Build history of the part. All positions in model axes, mm. Face numbers are marked on the shaded views. A direction names the side the tool comes from. Coordinates: 2 decimals unless noted, no trailing zeros. Write each loop counter-clockwise with the first axis right and the second up, starting at its lowest first coordinate (ties: lowest second). Pieces come first, ordered by that corner, then holes.
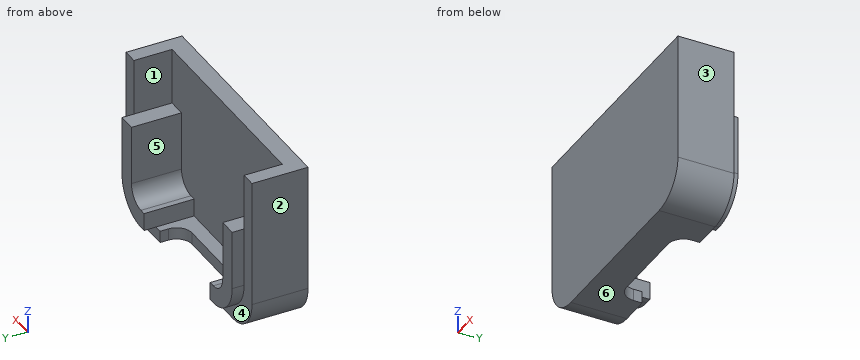
```python
from build123d import *

# Parameters (mm, degrees)
BOSS_EXTRUDE1_DEPTH = 1.5
BOSS_EXTRUDE2_START = 3.2
BOSS_EXTRUDE2_DEPTH = 3.2
BOSS_EXTRUDE3_START = 4.2
BOSS_EXTRUDE3_DEPTH = 4.2
CUT_EXTRUDE1_DEPTH  = 24.43560539


with BuildPart() as part:
    # Sketch1 → Boss-Extrude1 (new body)
    with BuildSketch(Plane(origin=(0, 0, 0), x_dir=(1, 0, 0), z_dir=(0, 1, 0))):
        with BuildLine():
            Line((-1.5, 20.46), (-1.5, 9.7))
            Line((-1.5, 9.7), (18.5, 9.7))
            Line((18.5, 9.7), (18.5, 20.46))
            ThreePointArc((18.5, 20.46), (17.621320344, 22.581320344), (15.5, 23.46))
            Line((15.5, 23.46), (1.5, 23.46))
            ThreePointArc((1.5, 23.46), (-0.621320344, 22.581320344), (-1.5, 20.46))
        make_face()
    extrude(amount=-BOSS_EXTRUDE1_DEPTH)

    # Sketch3 → Boss-Extrude2 (add)
    with BuildSketch(Plane(origin=(0, 0, 0), x_dir=(1, 0, 0), z_dir=(0, 1, 0)).offset(BOSS_EXTRUDE2_START)):
        with BuildLine():
            Line((2.75, 22.46), (14.25, 22.46))
            ThreePointArc((14.25, 22.46), (16.371320344, 21.581320344), (17.25, 19.46))
            Line((17.25, 19.46), (17.25, 9.7))
            Line((17.25, 9.7), (18.5, 9.7))
            Line((18.5, 9.7), (18.5, 20.46))
            ThreePointArc((18.5, 20.46), (17.621320344, 22.581320344), (15.5, 23.46))
            Line((15.5, 23.46), (1.5, 23.46))
            ThreePointArc((1.5, 23.46), (-0.621320344, 22.581320344), (-1.5, 20.46))
            Line((-1.5, 20.46), (-1.5, 9.7))
            Line((-1.5, 9.7), (-0.25, 9.7))
            Line((-0.25, 9.7), (-0.25, 19.46))
            ThreePointArc((-0.25, 19.46), (0.628679656, 21.581320344), (2.75, 22.46))
        make_face()
    extrude(amount=-BOSS_EXTRUDE2_DEPTH)

    # Sketch2 → Boss-Extrude3 (add)
    with BuildSketch(Plane(origin=(0, 0, 0), x_dir=(1, 0, 0), z_dir=(0, 1, 0)).offset(BOSS_EXTRUDE3_START)):
        with BuildLine():
            Line((2.75, 20.96), (3.25, 20.96))
            Line((3.25, 20.96), (3.25, 22.46))
            Line((3.25, 22.46), (2.75, 22.46))
            ThreePointArc((2.75, 22.46), (0.628679656, 21.581320344), (-0.25, 19.46))
            Line((-0.25, 19.46), (-0.25, 14.46))
            Line((-0.25, 14.46), (1.25, 14.46))
            Line((1.25, 14.46), (1.25, 19.46))
            ThreePointArc((1.25, 19.46), (1.689339828, 20.520660172), (2.75, 20.96))
        make_face()
        with BuildLine():
            Line((17.25, 19.46), (17.25, 14.46))
            Line((17.25, 14.46), (15.75, 14.46))
            Line((15.75, 14.46), (15.75, 19.46))
            ThreePointArc((15.75, 19.46), (15.310660172, 20.520660172), (14.25, 20.96))
            Line((14.25, 20.96), (13.75, 20.96))
            Line((13.75, 20.96), (13.75, 22.46))
            Line((13.75, 22.46), (14.25, 22.46))
            ThreePointArc((14.25, 22.46), (16.371320344, 21.581320344), (17.25, 19.46))
        make_face()
    extrude(amount=-BOSS_EXTRUDE3_DEPTH)

    # Sketch5 → Cut-Extrude1 (cut, through all)
    with BuildSketch(Plane(origin=(0, 0, -23.46), x_dir=(-1, 0, 0), z_dir=(0, 0, -1))):
        with BuildLine():
            Line((-13.1, 3.2), (-3.9, 3.2))
            Line((-3.9, 3.2), (-3.9, 2.5))
            ThreePointArc((-3.9, 2.5), (-4.280761184, 1.580761184), (-5.2, 1.2))
            Line((-5.2, 1.2), (-11.8, 1.2))
            ThreePointArc((-11.8, 1.2), (-12.719238816, 1.580761184), (-13.1, 2.5))
            Line((-13.1, 2.5), (-13.1, 3.2))
        make_face()
    extrude(amount=-CUT_EXTRUDE1_DEPTH, mode=Mode.SUBTRACT)


solid = part.part
```
1. Probe line 1 along X through (y, z) = (0.05, -16); line 2 along X through (y, z) = (1.85, -13); line 3 along Y through (x, z) = (10, -14). List the from-to ranges inside material, lowest first.
Computed values:
line 1: x = -1.5 to 1.25, 15.75 to 18.5
line 2: x = -1.5 to -0.25, 17.25 to 18.5
line 3: y = -1.5 to 0
2. Flat gauge pins, fed straight in: pin 1 (0.5 mm diameter, centred on x = 8.5, z = -23, fed in from +Y); pin 2 (1.2 mm diameter, centred on y = 2, z = -22, fed in from +X); pin 3 (1 mm diameter, centred on x = 11, z = -12, fed in from +Y). Where does each tip first touch, or does it go through?
Computed values:
pin 1: stops at y = 1.2
pin 2: stops at x = 18.35
pin 3: stops at y = 0
3. Saw through at C-C on x = 5.5. List the corners of the cut face in (y, z).
Computed values:
outline: (-1.5, -23.46) - (1.2, -23.46) - (1.2, -22.46) - (0, -22.46) - (0, -9.7) - (-1.5, -9.7) - close
4. Saw through at A-A on y = 2.8. List the corners of the cut face in (x, z).
Computed values:
outline: (-1.5, -20.46) arc R3 ccw to (1.5, -23.46) - (3.9, -23.46) - (3.9, -22.46) - (3.25, -22.46) - (3.25, -20.96) - (2.75, -20.96) arc R1.5 cw to (1.25, -19.46) - (1.25, -14.46) - (-0.25, -14.46) - (-0.25, -9.7) - (-1.5, -9.7) - close; (13.1, -23.46) - (15.5, -23.46) arc R3 ccw to (18.5, -20.46) - (18.5, -9.7) - (17.25, -9.7) - (17.25, -14.46) - (15.75, -14.46) - (15.75, -19.46) arc R1.5 cw to (14.25, -20.96) - (13.75, -20.96) - (13.75, -22.46) - (13.1, -22.46) - close
5. Saw through at D-D on y = 0.65. List the corners of the cut face in (x, z).
Computed values:
outline: (-1.5, -20.46) arc R3 ccw to (1.5, -23.46) - (15.5, -23.46) arc R3 ccw to (18.5, -20.46) - (18.5, -9.7) - (17.25, -9.7) - (17.25, -14.46) - (15.75, -14.46) - (15.75, -19.46) arc R1.5 cw to (14.25, -20.96) - (13.75, -20.96) - (13.75, -22.46) - (3.25, -22.46) - (3.25, -20.96) - (2.75, -20.96) arc R1.5 cw to (1.25, -19.46) - (1.25, -14.46) - (-0.25, -14.46) - (-0.25, -9.7) - (-1.5, -9.7) - close
6. Saw through at B-B on z = -19.25. List the corners of the cut face in (x, y), plus the area to 3 significant figures.
Computed values:
outline: (-1.5, -1.5) - (18.5, -1.5) - (18.5, 3.2) - (17.25, 3.2) - (17.25, 4.2) - (15.75, 4.2) - (15.75, 0) - (1.25, 0) - (1.25, 4.2) - (-0.25, 4.2) - (-0.25, 3.2) - (-1.5, 3.2) - close
area: 50.6 mm2
7. 3-axis set-ups, long thin cutter, end or side, ignore diameter. For the marked faces 4, 5 and 6: which of +Z, -Z, +X, -X, +Y, -Y reach the whole face in a straight line?
Computed values:
face 4: -Z, -X, +Y
face 5: +Z, +Y
face 6: -Z, +X, -X, +Y, -Y
8. Mould opens along X. For the marked faces 1, 2 and 3 say: +X half, -X half, draft (parallel to the pull), parting line (faces both ways), or undercut.
Computed values:
face 1: undercut
face 2: -X half
face 3: +X half
